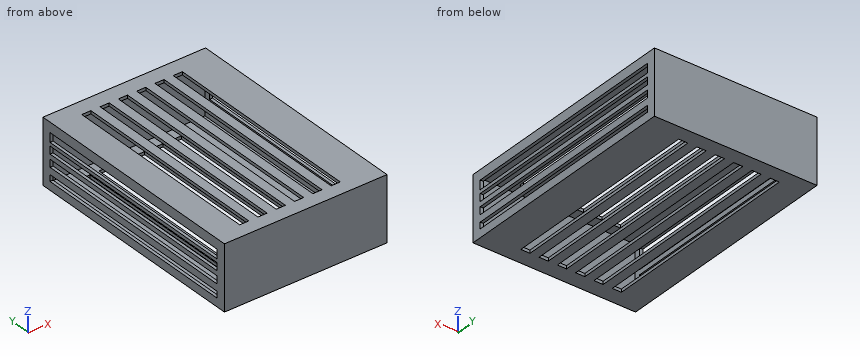
```python
from build123d import *

# Parameters (mm, degrees)
F0_W      = 213.36
F0_H      = 304.8
F0_W_2    = 205.36
F0_H_2    = 296.8
F1_DEPTH  = 4
F2_DEPTH  = 76.2
F3_W      = 213.36
F3_H      = 304.8
F3_W_2    = 205.36
F3_H_2    = 296.8
F4_DEPTH  = 4
F5_W      = 12
F5_H      = 265.28765991
F6_DEPTH  = 5.08
F7_W      = 12
F7_H      = 265.28765991
F8_DEPTH  = 5.08
F9_W      = 280.9167951345
F9_H      = 12.0694674551
F9_H_2    = 9.9573098123
F9_H_3    = 9.957306087
F9_H_4    = 8.4486240521
F10_DEPTH = 287.02


with BuildPart() as f1:
    # F0 (on Top) → F1 (new body)
    with BuildSketch(Plane.XY):
        Rectangle(F0_W, F0_H)
        Rectangle(F0_W_2, F0_H_2, mode=Mode.SUBTRACT)
        Rectangle(F0_W_2, F0_H_2)
    extrude(amount=-F1_DEPTH)

    # F0 (on Top) → F2 (join)
    with BuildSketch(Plane.XY):
        Rectangle(F0_W, F0_H)
        Rectangle(F0_W_2, F0_H_2, mode=Mode.SUBTRACT)
    extrude(amount=F2_DEPTH)

    # F3 (on face) → F4 (join)
    with BuildSketch(Plane.XY.offset(76.2)):
        Rectangle(F3_W, F3_H)
        Rectangle(F3_W_2, F3_H_2, mode=Mode.SUBTRACT)
        Rectangle(F3_W_2, F3_H_2)
    extrude(amount=F4_DEPTH)

    # F5 (on face) → F6 (cut)
    with BuildSketch(Plane.XY.offset(80.2)):
        with Locations((-66, -1.0106861591)):
            Rectangle(F5_W, F5_H)
        with Locations((-42, -1.0106861591)):
            Rectangle(F5_W, F5_H)
        with Locations((-18, -1.0106861591)):
            Rectangle(F5_W, F5_H)
        with Locations((6, -1.0106861591)):
            Rectangle(F5_W, F5_H)
        with Locations((30, -1.0106861591)):
            Rectangle(F5_W, F5_H)
        with Locations((54, -1.0106861591)):
            Rectangle(F5_W, F5_H)
    extrude(amount=-F6_DEPTH, mode=Mode.SUBTRACT)

    # F7 (on face) → F8 (cut)
    with BuildSketch(Plane(origin=(0, 0, -4), x_dir=(1, 0, 0), z_dir=(0, 0, -1))):
        with Locations((-66, -0.8343393173)):
            Rectangle(F7_W, F7_H)
        with Locations((-42, -0.8343393173)):
            Rectangle(F7_W, F7_H)
        with Locations((-18, -0.8343393173)):
            Rectangle(F7_W, F7_H)
        with Locations((6, -0.8343393173)):
            Rectangle(F7_W, F7_H)
        with Locations((30, -0.8343393173)):
            Rectangle(F7_W, F7_H)
        with Locations((54, -0.8343393173)):
            Rectangle(F7_W, F7_H)
    extrude(amount=-F8_DEPTH, mode=Mode.SUBTRACT)

    # F9 (on face) → F10 (cut)
    with BuildSketch(Plane(origin=(-106.68, 0, 0), x_dir=(0, -1, 0), z_dir=(-1, 0, 0))):
        with Locations((-0.1723989844, 61.221299693)):
            Rectangle(F9_W, F9_H)
        with Locations((-0.1723989844, 45.6818621606)):
            Rectangle(F9_W, F9_H_2)
        with Locations((-0.1723989844, 29.3880850077)):
            Rectangle(F9_W, F9_H_3)
        with Locations((-0.1723989844, 11.1330202781)):
            Rectangle(F9_W, F9_H_4)
    extrude(amount=-F10_DEPTH, mode=Mode.SUBTRACT)


solid = f1.part
```
The model under review builds one solid part; all positions refer to its coordinate system, in mm. Round coordinates to 2 decimals unless told otherwise and drop trailing zeros. Order: outer loops, then holes, each group sorted by start corner. A loop starts at its lowest first (then second) coordinate and runs counter-clockwise, first axis right, second up. Notation, with made-up numbers: (80.5, -30) -> (100.5, -30) arc R35 cw to (100.5, 6) -> close; hole circle Ø4 at (66.25, 11.5). An arc over 180 degrees is marked (long way). One line per item, written item: value. Start each with the question number.
Q1. Take a section at B-B (x = 91). Write out the cut boundary in (y, z).
Q2. Take a section at C-C (y = 15.5). Count the separate pieces of the cut face and the enclosed holes in it, and give its area (3 significant figures).
Q3. Wall thickness on line 1 (Y direction, x = -57.5, z = 25.5); line 2 (Z direction, x = 42, y = 60); line 3 (X direction, y = 22, z = 17): over which ranges is each line inside the solid? List them lowest first.
Q4. Take a section at A-A (z = 12). Write out the cut boundary in (x, y).
Reported:
1. outline: (-152.4, -4) -> (152.4, -4) -> (152.4, 80.2) -> (-152.4, 80.2) -> close; hole (-148.4, 0) -> (148.4, 0) -> (148.4, 76.2) -> (-148.4, 76.2) -> close
2. separate pieces: 20
2. enclosed holes: 0
2. area: 1,420 mm2
3. line 1: y = -152.4 to -148.4, 148.4 to 152.4
3. line 2: z = -4 to 0, 76.2 to 80.2
3. line 3: x = -106.68 to -102.68, 102.68 to 106.68
4. outline: (-106.68, -152.4) -> (106.68, -152.4) -> (106.68, -140.29) -> (102.68, -140.29) -> (102.68, -148.4) -> (-102.68, -148.4) -> (-102.68, -140.29) -> (-106.68, -140.29) -> close; (-106.68, 140.63) -> (-102.68, 140.63) -> (-102.68, 148.4) -> (102.68, 148.4) -> (102.68, 140.63) -> (106.68, 140.63) -> (106.68, 152.4) -> (-106.68, 152.4) -> close
